```python
from build123d import *

# Parameters (mm, degrees)
BOSS_EXTRUDE2_DEPTH = 3
FILLET1_R           = 1.5


with BuildPart() as part:
    # Sketch1 → Boss-Extrude2 (new body)
    with BuildSketch(Plane(origin=(0, 0, 0), x_dir=(1, 0, 0), z_dir=(0, 1, 0))):
        Polygon((0, 0), (70, 70), (130, 70), (60, 0), (55, 0), (55, -12.7), (5, -12.7), (5, 0), align=None)
    extrude(amount=BOSS_EXTRUDE2_DEPTH)

    # Fillet1
    fillet1_edges = [part.edges().sort_by_distance(p)[0] for p in [
        (35, 3, -35),
        (35, 0, -35),
    ]]
    fillet(fillet1_edges, radius=FILLET1_R - 0.0001)  # a hair under: the kernel refuses the full size


solid = part.part
```
Part model, mm, in its own coordinate system. A direction names the side the tool comes from. Coordinates: 2 decimals unless noted, no trailing zeros. Order: outer loops, then holes, each group sorted by start corner. A loop starts at its lowest first (then second) coordinate and runs counter-clockwise, first axis right, second up. Notation, with made-up numbers: (76, -3.5) - (100, -3.5) arc R6 cw to (100, 4.5) - close; hole circle Ø8 at (-35.75, -5.5). An arc over 180 degrees is marked (long way). Return JSON: item names as keys, results as strings. Group by question number.
Item 1: Which spindle directions (+Z, -Z, +X, -X, +Y, -Y) get a long thin tool onto all of the face, cutting with end or side? Do faces 1 (the face through (36.33, 0.451, -35.725)), 2 (the face through (55, 1, 6)), 3 (the face through (3, 1, 0)). Say none if no direction does.
Item 2: Pin check, flat tips, straight feed: pin 1 (1.5 mm diameter, centred on y = 1, z = -11, fed in from -X); pin 2 (6 mm diameter, centred on x = 51.5, z = -55, fed in from +Y); pin 3 (0.9 mm diameter, centred on x = 56.5, y = 1.5, fed in from +Z). Stop position of each tip, or through.
Item 3: Cut at A-A (y = 2.05). List the corners of the cut face in (x, z), plus the area to 3 significant figures.
Item 4: Cut at B-B (x = 92). List the corners of the cut face in (y, z), plus the area to 3 significant figures.
Item 5: Drill centre lines: probe 1 along Z at (x, y) = (11.5, 1.45); probe 2 along X at (y, z) = (1.8, -49); probe 3 along Z at (x, y) = (63, 0.7). Where is each one in solid material? Low to high. Write a range as from..to.
Item 6: Cut at C-C (x = 110). List the corners of the cut face in (y, z), plus the area to 3 significant figures.
Check values:
{
 "1": {"face 1": "-Z, -X, -Y", "face 2": "+Z, +X, +Y, -Y", "face 3": "+Z, -X, +Y, -Y"},
 "2": {"pin 1": "stops at x = 10.32", "pin 2": "stops at y = 2.64", "pin 3": "stops at z = 0"},
 "3": {"outline": "(0.15, 0) - (70.15, -70) - (130, -70) - (60, 0) - (55, 0) - (55, 12.7) - (5, 12.7) - (5, 0) - close", "area": "4,820 mm2"},
 "4": {"outline": "(0, -70) - (3, -70) - (3, -32) - (0, -32) - close", "area": "114 mm2"},
 "5": {"probe 1": "z = -11.5..12.7", "probe 2": "x = 49.04..109", "probe 3": "z = -62.67..-3"},
 "6": {"outline": "(0, -70) - (3, -70) - (3, -50) - (0, -50) - close", "area": "60.0 mm2"}
}
